```python
from build123d import *

# Parameters (mm, degrees)
F1_DEPTH     = 3
F3_DEPTH     = 5
F5_DEPTH     = 3
F6_T3_DEPTH  = 28
F6_T5_DEPTH  = 24
F6_T7_DEPTH  = 2
F6_T10_ANGLE = 180
F6_T12_ANGLE = 90
F6_T14_ANGLE = 90
F6_T16_ANGLE = 90
F6_T18_ANGLE = 90
F6_T20_ANGLE = 180


# Not quite as in the source:
# - a fillet or chamfer that OpenCascade refuses, or shapes differently, is made with other operations: its cross-section is extruded or revolved along the edge and cut away or added


with BuildPart() as f1:
    # F0 (on Front) → F1 (new body)
    with BuildSketch(Plane.XZ):
        with BuildLine():
            Line((29, 13), (5, 13))
            ThreePointArc((5, 13), (1.4644660941, 11.5355339059), (0, 8))
            Line((0, 8), (0, -20))
            ThreePointArc((0, -20), (1.4644660941, -23.5355339059), (5, -25))
            Line((5, -25), (29, -25))
            ThreePointArc((29, -25), (32.5355339059, -23.5355339059), (34, -20))
            Line((34, -20), (34, 8))
            ThreePointArc((34, 8), (32.5355339059, 11.5355339059), (29, 13))
        make_face()
    extrude(amount=F1_DEPTH)

    # F2 (on face) → F3 (join)
    with BuildSketch(Plane.XZ.offset(3)):
        with BuildLine():
            ThreePointArc((14.5, 0), (17, -2.5), (19.5, 0))
            ThreePointArc((19.5, 0), (17, 2.5), (14.5, 0))
        make_face()
    extrude(amount=F3_DEPTH)

    # F4 (on face) → F5 (join)
    with BuildSketch(Plane.XZ.offset(8)):
        with BuildLine():
            Line((19.5, 0), (19.5, 2))
            ThreePointArc((19.5, 2), (17, 4.5), (14.5, 2))
            Line((14.5, 2), (14.5, 0))
            ThreePointArc((14.5, 0), (17, -2.5), (19.5, 0))
        make_face()
    extrude(amount=F5_DEPTH)

    # F6: fillet of radius 2.5 on 13 edges, made by hand

    # F6_s1 → F6_t2 (revolve)
    with BuildSketch(Plane.XY):
        with BuildLine():
            ThreePointArc((12, -3), (13.767766953, -3.732233047), (14.5, -5.5))
            Line((14.5, -5.5), (14.5, -3))
            Line((14.5, -3), (12, -3))
        make_face()
    revolve(axis=Axis((17, -3, 0), (0, -1, 0)))

    # F6_s4 → F6_t3 (cut)
    with BuildSketch(Plane.XY.offset(-20)):
        with BuildLine():
            ThreePointArc((34, -0.5), (33.267766953, -2.267766953), (31.5, -3))
            Line((31.5, -3), (34, -3))
            Line((34, -3), (34, -0.5))
        make_face()
        with BuildLine():
            ThreePointArc((2.5, -3), (0.732233047, -2.267766953), (0, -0.5))
            Line((0, -0.5), (0, -3))
            Line((0, -3), (2.5, -3))
        make_face()
    extrude(amount=F6_T3_DEPTH, mode=Mode.SUBTRACT)

    # F6_s6 → F6_t5 (cut)
    with BuildSketch(Plane.YZ.offset(5)):
        with BuildLine():
            ThreePointArc((-3, -22.5), (-2.267766953, -24.267766953), (-0.5, -25))
            Line((-0.5, -25), (-3, -25))
            Line((-3, -25), (-3, -22.5))
        make_face()
        with BuildLine():
            ThreePointArc((-3, 10.5), (-2.267766953, 12.267766953), (-0.5, 13))
            Line((-0.5, 13), (-3, 13))
            Line((-3, 13), (-3, 10.5))
        make_face()
    extrude(amount=F6_T5_DEPTH, mode=Mode.SUBTRACT)

    # F6_s8 → F6_t7 (cut)
    with BuildSketch(Plane.XY):
        with BuildLine():
            ThreePointArc((19.5, -8.5), (18.767766953, -10.267766953), (17, -11))
            Line((17, -11), (19.5, -11))
            Line((19.5, -11), (19.5, -8.5))
        make_face()
        with BuildLine():
            ThreePointArc((17, -11), (15.232233047, -10.267766953), (14.5, -8.5))
            Line((14.5, -8.5), (14.5, -11))
            Line((14.5, -11), (17, -11))
        make_face()
    extrude(amount=F6_T7_DEPTH, mode=Mode.SUBTRACT)

    # F6_s9 → F6_t10 (revolve, cut)
    with BuildSketch(Plane.XY):
        with BuildLine():
            ThreePointArc((14.5, -8.5), (15.232233047, -10.267766953), (17, -11))
            Line((17, -11), (14.5, -11))
            Line((14.5, -11), (14.5, -8.5))
        make_face()
    revolve(axis=Axis((17, -11, 0), (0, -1, 0)), revolution_arc=F6_T10_ANGLE, mode=Mode.SUBTRACT)

    # F6_s11 → F6_t12 (revolve, cut)
    with BuildSketch(Plane.YZ.offset(29)):
        with BuildLine():
            ThreePointArc((-0.5, -25), (-2.267766953, -24.267766953), (-3, -22.5))
            Line((-3, -22.5), (-3, -25))
            Line((-3, -25), (-0.5, -25))
        make_face()
    revolve(axis=Axis((29, -3, -20), (0, -1, 0)), revolution_arc=F6_T12_ANGLE, mode=Mode.SUBTRACT)

    # F6_s13 → F6_t14 (revolve, cut)
    with BuildSketch(Plane.XY.offset(8)):
        with BuildLine():
            ThreePointArc((34, -0.5), (33.267766953, -2.267766953), (31.5, -3))
            Line((31.5, -3), (34, -3))
            Line((34, -3), (34, -0.5))
        make_face()
    revolve(axis=Axis((29, -3, 8), (0, -1, 0)), revolution_arc=F6_T14_ANGLE, mode=Mode.SUBTRACT)

    # F6_s15 → F6_t16 (revolve, cut)
    with BuildSketch(Plane.XY.offset(-20)):
        with BuildLine():
            ThreePointArc((2.5, -3), (0.732233047, -2.267766953), (0, -0.5))
            Line((0, -0.5), (0, -3))
            Line((0, -3), (2.5, -3))
        make_face()
    revolve(axis=Axis((5, -3, -20), (0, -1, 0)), revolution_arc=F6_T16_ANGLE, mode=Mode.SUBTRACT)

    # F6_s17 → F6_t18 (revolve, cut)
    with BuildSketch(Plane.YZ.offset(5)):
        with BuildLine():
            ThreePointArc((-3, 10.5), (-2.267766953, 12.267766953), (-0.5, 13))
            Line((-0.5, 13), (-3, 13))
            Line((-3, 13), (-3, 10.5))
        make_face()
    revolve(axis=Axis((5, -3, 8), (0, -1, 0)), revolution_arc=F6_T18_ANGLE, mode=Mode.SUBTRACT)

    # F6_s19 → F6_t20 (revolve, cut)
    with BuildSketch(Plane.XY.offset(2)):
        with BuildLine():
            ThreePointArc((17, -11), (18.767766953, -10.267766953), (19.5, -8.5))
            Line((19.5, -8.5), (19.5, -11))
            Line((19.5, -11), (17, -11))
        make_face()
    revolve(axis=Axis((17, -11, 2), (0, -1, 0)), revolution_arc=F6_T20_ANGLE, mode=Mode.SUBTRACT)


solid = f1.part
```
Read the model definition and answer for the solid it produces. Units are mm, in the model's axes. A direction names the side the tool comes from. Give positions to 0.01 mm unless a question says otherwise; leave off trailing zeros. Write each loop counter-clockwise with the first axis right and the second up, starting at its lowest first coordinate (ties: lowest second). Pieces come first, ordered by that corner, then holes. Notation, with made-up numbers: M -6.75,-28 L 47.25,-28 A29 ccw 47.25,-4 Z; hole C 4,-35.75 d7. An arc over 180 degrees is marked long. Put each result on its own line as item: value. Start each with the question number.
1. For a pull along Y with two mould halves and no side action, classify faces 3 (the cylindrical face through (0.752, -2.287, -6.196)), 4 (the flat face through (17, -8, 3)), 5 (the cylindrical face through (16.46, -6.98, -2.44)), 6 (the cylindrical face through (1.5, -0.25, 11.57)) as released by +Y, released by -Y, zero draft, split by the parting line, or undercut.
2. The part is cut by section D-D, the plane y = -9. Give the vertices of the cut face in (x, z).
3. Consider line 1 along Y through (x, z) = (11, -8.5); line 2 along X through (y, z) = (-5.5, 0); line 3 along Y through (x, z) = (19, -2). Determine where each line is inside the solid, lowest interval first.
4. The part is cut by section B-B, the plane z = -6. Give the vertices of the cut face in (x, y), and give its area (3 significant figures).
5. Which of the six approach directions +Z, -Z, +X, -X, +Y, -Y give full straight-line access (tool end or side, diameter ignored) to faces 1 (the cylindrical face through (1.43, -0.25, -23.5)), 2 (the cylindrical face through (17.1, -8.2, 4.5))?
6. The part is cut by section C-C, the plane y = -1. Give the vertices of the cut face in (x, z), and give its area (3 significant figures).
7. The part is cut by section A-A, the plane x = 25.5. Give the vertices of the cut face in (y, z), and give its area (3 significant figures).
8. Each of these flat-tipped pins is pushed along its axis until it touches: pin 1 Ø12 at (x, z) = (11.5, -19) entering from -Y; pin 2 Ø3 at (y, z) = (-2.5, -14) entering from -X; pin 3 Ø1.5 at (x, y) = (6, -3) entering from +Z. Where does it stop, or does it pass through?
Final values:
1. face 3: released by -Y
1. face 4: undercut
1. face 5: undercut
1. face 6: zero draft
2. outline: M 14.55,0 A2.45 ccw 19.45,0 L 19.45,2 A2.45 ccw 14.55,2 Z
3. line 1: y = -3 to 0
3. line 2: x = 14.5 to 19.5
3. line 3: y = -4.26 to 0
4. outline: M 0,-0.5 A2.5 ccw 2.5,-3 L 31.5,-3 A2.5 ccw 34,-0.5 L 34,0 L 0,0 Z
4. area: 99.3 mm²
5. face 1: -Z, -X, +Y, -Y
5. face 2: +Z, -Y
6. outline: M 0.05,-20 A4.95 ccw 5,-24.95 L 29,-24.95 A4.95 ccw 33.95,-20 L 33.95,8 A4.95 ccw 29,12.95 L 5,12.95 A4.95 ccw 0.05,8 Z
6. area: 1,260 mm²
7. outline: M -3,-22.5 A2.5 ccw -0.5,-25 L 0,-25 L 0,13 L -0.5,13 A2.5 ccw -3,10.5 Z
7. area: 111 mm²
8. pin 1: stops at y = -3
8. pin 2: stops at x = 0.05
8. pin 3: stops at z = 12.29
